```python
from build123d import *

# Parameters (mm, degrees)
SKETCH1_R           = 130.175
SKETCH1_R_2         = 128.525
BOSS_EXTRUDE1_DEPTH = 234.95
SKETCH2_R           = 130.175
BOSS_EXTRUDE2_DEPTH = 1.65
SKETCH3_R           = 3.96875
CUT_EXTRUDE1_DEPTH  = 237.6


with BuildPart() as part:
    # Sketch1 → Boss-Extrude1 (new body)
    with BuildSketch(Plane(origin=(0, 0, 0), x_dir=(1, 0, 0), z_dir=(0, 1, 0))):
        Circle(SKETCH1_R)
        Circle(SKETCH1_R_2, mode=Mode.SUBTRACT)
    extrude(amount=BOSS_EXTRUDE1_DEPTH)

    # Sketch2 → Boss-Extrude2 (add)
    with BuildSketch(Plane.XZ):
        Circle(SKETCH2_R)
    extrude(amount=BOSS_EXTRUDE2_DEPTH)

    # Sketch3 → Cut-Extrude1 (cut, through all)
    with BuildSketch(Plane.XZ.offset(1.65)):
        Circle(SKETCH3_R)
    extrude(amount=-CUT_EXTRUDE1_DEPTH, mode=Mode.SUBTRACT)


solid = part.part
```
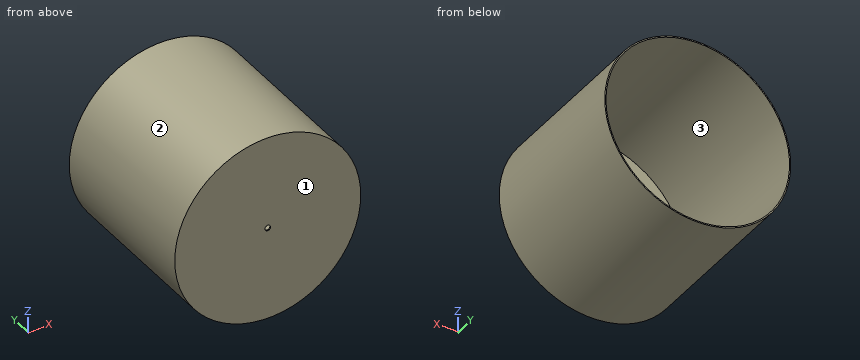
Input: part model. Units: mm. Frame: model coordinates. Face numbers are marked on the shaded views. Give positions to 0.01 mm unless a question says otherwise; leave off trailing zeros. Order: outer loops, then holes, each group sorted by start corner. A loop starts at its lowest first (then second) coordinate and runs counter-clockwise, first axis right, second up.
1. Material intervals for L1, parallel to Z at x = 0, y = -0.75 (3 decimals); L2, parallel to Z at x = 0, y = 60.5 (3 decimals), sorted ascending.
Derived:
L1: z = -130.175 to -3.969, 3.969 to 130.175
L2: z = -130.175 to -128.525, 128.525 to 130.175
2. Section C-C on y = 166. Return the cut outline in (x, z) (3 decimals).
Derived:
outline: circle Ø260.35 at (0, 0); hole circle Ø257.05 at (0, 0)
3. Section D-D on z = -66.5. Return the cut outline in (x, y), and give its area (3 significant figures).
Derived:
outline: (-111.91, -1.65) - (111.91, -1.65) - (111.91, 234.95) - (109.98, 234.95) - (109.98, 0) - (-109.98, 0) - (-109.98, 234.95) - (-111.91, 234.95) - close
area: 1,270 mm2
4. Pin query (flat end, axial travel): pin 1 (3 mm diameter, centred on y = 82.5, z = -18, fed in from +X); pin 2 (2 mm diameter, centred on x = -50.5, z = 50, fed in from +Y); pin 3 (1 mm diameter, centred on y = 200, z = 32.5, fed in from -X). Return the tip coordinate at first contact, or that it passes through.
Derived:
pin 1: stops at x = 129.13
pin 2: stops at y = 0
pin 3: stops at x = -126.18
5. Mould query, pull axis X, two halves, no side actions, for the marked faces 1, 2 and 3. Classes: released by +X, released by -X, zero draft, split by the parting line, or undercut.
Derived:
face 1: zero draft
face 2: split by the parting line
face 3: undercut
6. Section A-A on z = 0. Return the cut outline in (x, y) (3 decimals), and give its area (3 significant figures).
Derived:
outline: (-130.175, -1.65) - (-3.969, -1.65) - (-3.969, 0) - (-128.525, 0) - (-128.525, 234.95) - (-130.175, 234.95) - close; (3.969, -1.65) - (130.175, -1.65) - (130.175, 234.95) - (128.525, 234.95) - (128.525, 0) - (3.969, 0) - close
area: 1,190 mm2
7. Section B-B on x = 0. Return the cut outline in (y, z) (3 decimals).
Derived:
outline: (-1.65, -130.175) - (234.95, -130.175) - (234.95, -128.525) - (0, -128.525) - (0, -3.969) - (-1.65, -3.969) - close; (-1.65, 3.969) - (0, 3.969) - (0, 128.525) - (234.95, 128.525) - (234.95, 130.175) - (-1.65, 130.175) - close
